```python
from build123d import *

# Parameters (mm, degrees)
SKETCH1_W                = 4
SKETCH1_H                = 12
EXTRUDE_THIN2_DEPTH      = 0.5
FILLET2_R                = 1
CIRPATTERN1_COUNT        = 3
FILLET2_OF_CIRPATTERN1_R = 1


with BuildPart() as part:
    # Sketch1 → Extrude-Thin2 (new body)
    with BuildSketch(Plane.YZ):
        with Locations((0, 6)):
            Rectangle(SKETCH1_W, SKETCH1_H)
    extrude_thin2 = extrude(amount=EXTRUDE_THIN2_DEPTH)

    # Fillet2
    fillet2_edges = [part.edges().sort_by_distance(p)[0] for p in [
        (0.25, -2, 12),
        (0.25, 2, 12),
    ]]
    fillet(fillet2_edges, radius=FILLET2_R)

    # CirPattern1: Extrude-Thin2 ×3 about axis
    cirpattern1_axis = Axis((0, 0, 0), (1, 0, 0))
    for i in range(1, CIRPATTERN1_COUNT):
        add(extrude_thin2.rotate(cirpattern1_axis, i * 360 / CIRPATTERN1_COUNT))

    # Fillet2 of CirPattern1
    fillet2_of_cirpattern1_edges = [part.edges().sort_by_distance(p)[0] for p in [
        (0.25, -9.392304845, -7.732050808),
        (0.25, -11.392304845, -4.267949192),
        (0.25, 11.392304845, -4.267949192),
        (0.25, 9.392304845, -7.732050808),
    ]]
    fillet(fillet2_of_cirpattern1_edges, radius=FILLET2_OF_CIRPATTERN1_R)


solid = part.part
```
Here's how the part is built. I have some questions about the finished solid (model axes, mm). A direction names the side the tool comes from. Give positions to 0.01 mm unless a question says otherwise; leave off trailing zeros. Loops run counter-clockwise (first coordinate to the right, second up) from the corner with the lowest first, then second, coordinate; pieces in that order, holes last. Notation, with made-up numbers: (55, -37.75) -> (85, -37.75) arc R22 cw to (85, -23.75) -> close; hole circle Ø11 at (63, 45.5). An arc over 180 degrees is marked (long way). Use one line per item in the form item = value. Start each with the question number.
1) Thinking about a two-plate mould opening in Y: for faces 3 (the face through (0.25, 10.4, -5.99)), 4 (the face through (0.254, -1.715, 11.699)), 5 (the face through (0, 0, 0)), 6 (the face through (0.246, -4.203, -4.736)), which applies, +Y half, -Y half, draft (parallel to the pull), parting line (faces both ways), or undercut?
2) For P1, Ø2, axis at y = -3.5, z = -2.5, coming from the -X side, with a flat end and sliding along its axis, tell me the tip position at first contact or that it passes through.
3) Which directions (+Z, -Z, +X, -X, +Y, -Y) give clear straight access to the entire face, cutting with the end or side of a thin tool? Please do faces 1 (the face through (0.25, -6.2, -1.27)), 2 (the face through (0.246, 4.203, -4.736)).
4) Imagine slicing it at C-C (z = 4.5). Please give me the cut outline in (x, y).
5) Imagine slicing it at B-B (z = -2.75). Please give me the cut outline in (x, y).
6) Imagine slicing it at D-D (y = 0.5). Please give me the cut outline in (x, z).
7) Please list where these lines run through material, in increasing order: line 1 along Y through (x, z) = (0.05, 7); line 2 along Z through (x, y) = (0.25, 3.5); line 3 along Z through (x, y) = (0.15, 7.25).
8) Imagine slicing it at A-A (x = 0.1). Please give me the cut outline in (y, z), then the cut area to 3 significant figures.
Check values:
q1.face_3 = +Y half
q1.face_4 = -Y half
q1.face_5 = draft
q1.face_6 = undercut
q2.P1 = 0
q3.face_1 = +Z, +X, -X, -Y
q3.face_2 = -Z, +X, -X
q4.outline = (0, -2) -> (0.5, -2) -> (0.5, 2) -> (0, 2) -> close
q5.outline = (0, -8.76) -> (0.5, -8.76) -> (0.5, -0.76) -> (0, -0.76) -> close; (0, 0.76) -> (0.5, 0.76) -> (0.5, 8.76) -> (0, 8.76) -> close
q6.outline = (0, -2.6) -> (0.5, -2.6) -> (0.5, 12) -> (0, 12) -> close
q7.line_1 = -2 to 2
q7.line_2 = -4.33 to 0.29
q7.line_3 = -6.5 to -1.88
q8.outline = (-10.89, -5.13) -> (-9.89, -6.87) arc R1 ccw to (-8.53, -7.23) -> (0, -2.31) -> (8.53, -7.23) arc R1 ccw to (9.89, -6.87) -> (10.89, -5.13) arc R1 ccw to (10.53, -3.77) -> (2, 1.15) -> (2, 11) arc R1 ccw to (1, 12) -> (-1, 12) arc R1 ccw to (-2, 11) -> (-2, 1.15) -> (-10.53, -3.77) arc R1 ccw to start
q8.area = 136 mm^2
